Geometry check sheet. Reference: the model listing, model coordinates, mm. A direction names the side the tool comes from. Give positions to 0.01 mm unless a question says otherwise; leave off trailing zeros. Order: outer loops, then holes, each group sorted by start corner. A loop starts at its lowest first (then second) coordinate and runs counter-clockwise, first axis right, second up. Notation, with made-up numbers: M 21.5,40 L 69.5,40 A20 cw 69.5,48 Z; hole C 54.25,67.5 d2. An arc over 180 degrees is marked long. Answer as CSV lines item,"result".
from build123d import *

# Parameters (mm, degrees)
F1_W     = 482.6
F1_H     = 88.9
F2_DEPTH = 1.5875
F3_W     = 444.5
F3_H     = 88.9
F4_DEPTH = 226.06


# Not quite as in the source:
# - a variable given as a bare number and used for a length is read in inches; the dataset says mm whatever the document's units were


with BuildPart() as f2:
    # F1 (on Front) → F2 (new body)
    with BuildSketch(Plane.XZ):
        Rectangle(F1_W, F1_H)
        with BuildLine():
            Line((-235.1024, -34.925), (-230.0224, -34.925))
            ThreePointArc((-230.0224, -34.925), (-226.8474, -38.1), (-230.0224, -41.275))
            Line((-230.0224, -41.275), (-235.1024, -41.275))
            ThreePointArc((-235.1024, -41.275), (-238.2774, -38.1), (-235.1024, -34.925))
        make_face(mode=Mode.SUBTRACT)
        with BuildLine():
            Line((230.0224, -34.925), (235.1024, -34.925))
            ThreePointArc((235.1024, -34.925), (238.2774, -38.1), (235.1024, -41.275))
            Line((235.1024, -41.275), (230.0224, -41.275))
            ThreePointArc((230.0224, -41.275), (226.8474, -38.1), (230.0224, -34.925))
        make_face(mode=Mode.SUBTRACT)
        with BuildLine():
            ThreePointArc((-235.1024, 34.925), (-238.2774, 38.1), (-235.1024, 41.275))
            Line((-235.1024, 41.275), (-230.0224, 41.275))
            ThreePointArc((-230.0224, 41.275), (-226.8474, 38.1), (-230.0224, 34.925))
            Line((-230.0224, 34.925), (-235.1024, 34.925))
        make_face(mode=Mode.SUBTRACT)
        with BuildLine():
            Line((235.1024, 34.925), (230.0224, 34.925))
            ThreePointArc((230.0224, 34.925), (226.8474, 38.1), (230.0224, 41.275))
            Line((230.0224, 41.275), (235.1024, 41.275))
            ThreePointArc((235.1024, 41.275), (238.2774, 38.1), (235.1024, 34.925))
        make_face(mode=Mode.SUBTRACT)
    extrude(amount=F2_DEPTH)

    # F3 (on face) → F4 (join)
    with BuildSketch(Plane(origin=(0, 0, 0), x_dir=(-1, 0, 0), z_dir=(0, 1, 0))):
        Rectangle(F3_W, F3_H)
    extrude(amount=F4_DEPTH)


solid = f2.part
(1) Section check A-A on z = 28. Enter the section's corners in (x, y), then the cut area to 3 significant figures.
The answers:
outline,"M -241.3,-1.59 L 241.3,-1.59 L 241.3,0 L 222.25,0 L 222.25,226.06 L -222.25,226.06 L -222.25,0 L -241.3,0 Z"
area,"101,000 mm2"
(2) Material ranges on line 1 (X direction, y = 115, z = -30), recorded low to high.
The answers:
line 1,"x = -222.25 to 222.25"
(3) Section check B-B on y = 81. Enter the section's corners in (x, z).
The answers:
outline,"M -222.25,-44.45 L 222.25,-44.45 L 222.25,44.45 L -222.25,44.45 Z"
(4) Tool access check on faces 1 (the face through (-222.25, 111, -1)), 2 (the face through (-3, -1.588, 1)), 3 (the face through (222.25, 111, -1)). Record the directions out of +Z, -Z, +X, -X, +Y, -Y that give a thin tool (end or side, any length) a straight path to the whole face; none if there is none.
The answers:
face 1,"+Z, -Z, -X, +Y"
face 2,"+Z, -Z, +X, -X, -Y"
face 3,"+Z, -Z, +X, +Y"
(5) Gauge pin test, flat ends, axial feed: P1, Ø15, axis at x = -232.5, z = -7, coming from the +Y side; P2, Ø1, axis at y = 202.5, z = -12, coming from the +X side. Record the tip position at first contact, or that the pin passes through.
The answers:
P1,"stops at y = 0"
P2,"stops at x = 222.25"
